Autodesk Fusion 360 part; units mm, degrees
sketch "Sketch1" plane through (0, 0, 0) normal (0, 1, 0) x (1, 0, 0)
  circle A0 centre (0, 0) radius 48 construction
  circle A1 centre (0, 0) radius 14 construction
  circle A2 centre (0, 0) radius 9.5 construction
  circle A3 centre (0, 0) radius 8 construction
  line L0 (0, 0) -> (8, 0) construction
  line L1 (0, 0) -> (0, -9.5) construction
  line L2 (0, 0) -> (-8, 0) construction
  line L3 (0, 0) -> (0, 9.5) construction
  circle A4 centre (8, 0) radius 1.5
  circle A5 centre (-8, 0) radius 1.5
  circle A6 centre (0, 9.5) radius 1.5
  circle A7 centre (0, 0) radius 12 construction
  line L4 (8, 0) -> (18, 0) construction
  line L5 (21.1, 0) -> (19.55, 2.6847) construction
  line L6 (19.55, 2.6847) -> (16.45, 2.6847) construction
  line L7 (16.45, 2.6847) -> (14.9, 0) construction
  line L8 (14.9, 0) -> (16.45, -2.6847) construction
  line L9 (16.45, -2.6847) -> (19.55, -2.6847) construction
  line L10 (19.55, -2.6847) -> (21.1, 0) construction
  circle A8 centre (18, 0) radius 3.1 construction
  circle A9 centre (18, 0) radius 1.5
  line L11 (0, 52) -> (-68, 52) construction
  line L12 (-9.7468, 47) -> (-68, 47) construction
  line L13 (-68, 52) -> (-68, 47) construction
  line L14 (-68, 47) -> (-68, 35.633) construction
  line L15 (-68, 35.633) -> (-32.1604, 35.633) construction
  line L16 (-68, 35.633) -> (-68, 30.833) construction
  line L17 (-68, 30.833) -> (-36.7876, 30.833) construction
  line L18 (-68, 30.833) -> (-68, -9.167) construction
  line L19 (-60, -9.167) -> (-47.1165, -9.167)
  line L20 (-68, -9.167) -> (-68, -13.967) construction
  line L21 (-68, -13.967) -> (-45.923, -13.967) construction
  line L22 (-60, -13.967) -> (-60, 35.633)
  line L23 (5.9333, 10.4305) -> (19.5328, 2.6945)
  line L24 (-60, -13.967) -> (21.1, -13.967)
  line L25 (21.1, -13.967) -> (21.1, 0)
  arc A10 (21.1, 0) -> (19.5328, 2.6945) centre (18, 0) ccw
  line L26 (-57, 35.633) -> (5, 35.633)
  line L27 (5, 35.633) -> (5, 11.8322)
  arc A11 (5.9333, 10.4305) -> (5.7778, 10.5175) centre (0, 0) ccw
  arc A12 (5, 11.8322) -> (5.7778, 10.5175) centre (6.5, 11.8322) ccw
  arc A13 (5.7778, 10.5175) -> (7.9656, 11.513) centre (6.5, 11.8322) ccw construction
  arc A14 (5.4445, 12.898) -> (5, 11.8322) centre (6.5, 11.8322) ccw construction
  arc A15 (7.9656, 11.513) -> (5.4445, 12.898) centre (6.5, 11.8322) ccw construction
  line L28 (5, 11.8322) -> (5, 10.9087) construction
  arc A16 (5.7778, 10.5175) -> (5, 10.9087) centre (0, 0) ccw construction
  line L29 (-57, 30.833) -> (5, 30.833)
  line L30 (-47.1165, -9.167) -> (21.1, -9.167)
  line L31 (-60, 35.633) -> (-60, 45.633)
  line L32 (-60, 45.633) -> (5, 45.633)
  line L33 (5, 45.633) -> (5, 35.633)
  circle A17 centre (-56, 42) radius 1.5
  circle A18 centre (-40, 42) radius 1.5
  line L34 (-40, 42) -> (0, 0) construction
  circle A19 centre (-55.8448, -4.167) radius 1.5
  line L35 (0, 0) -> (-55.8448, -4.167) construction
  line L36 (-68, -9.167) -> (-60, -9.167) construction
  line L37 (-57, -9.167) -> (-60, -8.167)
  line L38 (-57, -9.167) -> (-57, 30.833) construction
  line L39 (-57, 30.833) -> (-57, 35.633) construction
  line L40 (-57, 30.833) -> (-60, 29.833)
  line L41 (-57, 35.633) -> (-60, 36.633)
  line L42 (-60, 35.633) -> (-57, 35.633) construction
  line L43 (-60, 30.833) -> (-57, 30.833) construction
  line L44 (5, 11.8322) -> (5, -13.967) construction
  line L45 (5, -13.967) -> (19.8959, -2.4527)
  line L46 (18, 0) -> (19.8959, -2.4527) construction
  line L47 (18, 0) -> (21.1, 0) construction
  arc A20 (19.8959, -2.4527) -> (21.1, 0) centre (18, 0) ccw
  point P0 (18, 0)
  point P1 (-33.1034, 34.7586)
  point P2 (-47.8669, -3.5717)
  dimension "d1" = 96
  dimension "d2" = 28
  dimension "d3" = 19
  dimension "d4" = 16
  dimension "d5" = 3
  dimension "d6" = 3
  dimension "d7" = 3
  dimension "d8" = 24
  dimension "d9" = 18
  dimension "d10" = 3.1
  dimension "d11" = 60
  dimension "d12" = 3
  dimension "d13" = 52
  dimension "d14" = 68
  dimension "d15" = 68
  dimension "d18" = 5
  dimension "d22" = 16.367
  dimension "d23" = 4.8
  dimension "d24" = 40
  dimension "d25" = 4.8
  dimension "d26" = 8
  dimension "d27" = 3.1
  dimension "d28" = 5
  dimension "d33" = 12
  dimension "d34" = 3
  dimension "d35" = 10
  dimension "d36" = 3
  dimension "d37" = 12
  dimension "d38" = 5
  dimension "d39" = 3
  dimension "d40" = 5
  dimension "d41" = 10
  dimension "d42" = 3
  dimension "d43" = 5
  dimension "d44" = 8
  dimension "d54" = 1
  dimension "d55" = 3
  dimension "d56" = 1
  dimension "d57" = 1
  dimension "d60" = 3.1
extrude "Extrude1" add sketch "Sketch1" along normal blind 4.8 contours L19 L22 L37 | L19 L22 L24 L30 L45 | L19 L22 L23 A10 L27 A11 A12 L29 L30 L37 L40 L45 A20 | L22 L26 L27 L29 L31 L40 L41 | L26 L31 L32 L33 L41 makes body 1
fillet "Fillet1" radius 4 2 edges at (5, 2.4, -45.633) (-60, 2.4, -45.633) on bodies 1
extrude "Extrude2" cut sketch "Sketch1" along normal blind 1.8 contours L19 L22 L37 | L19 L22 L24 L30 L45 | L24 L25 L30 L45 | L22 L26 L27 L29 L31 L40 L41 bodies 1
fillet "Fillet2" radius 3 3 edges at (-57, 0.9, -35.633) (-57, 0.9, -30.833) (-57, 0.9, 9.167) on bodies 1
ref_plane "WorkPlane1" through (-30, 0, 0) normal (1, 0, 0) x (0, 1, 0)
ref_plane "WorkPlane2" through (-25, 0, 0) normal (1, 0, 0) x (0, 1, 0)
split "Split1" by plane through (-30, 0, 0) normal (1, 0, 0) bodies 1 makes body 2 at (-9.9784, 4.8, -33.9796)
split "Split2" by plane through (-25, 0, 0) normal (1, 0, 0) bodies 2 makes body 3 at (-8.25, 4.8, -34.0217)
delete_body "RemoveBody1" bodies 2
move_body "Move1" bodies 3 to x (1, 0, 0) y (0, 1, 0) z (0, 0, 1) at (-5, 0, 0)
combine "Combine1" operation add target body 1 tool bodies 3
Verification items for the finished model (mm, model axes). A direction names the side the tool comes from. Round coordinates to 2 decimals unless told otherwise and drop trailing zeros. Write each loop counter-clockwise with the first axis right and the second up, starting at its lowest first coordinate (ties: lowest second). Pieces come first, ordered by that corner, then holes.
(1) Mould release check, pull along X, two halves, no side actions. Record for faces 5 (the cylindrical face through (11.5, 2.37, 0.07)), 6 (the flat face through (-30, 0, -41)), 7 (the flat face through (-60, 2, -13)), 8 (the cylindrical face through (-1.14, 2.43, -44.43)): pulls with the +X half, pulls with the -X half, needs draft (parallel to the pull), parting line crosses it, or undercut.
Returned:
face 5: undercut
face 6: needs draft
face 7: pulls with the -X half
face 8: pulls with the +X half
(2) Section check C-C (x = -45.5). Enter the section's corners in (y, z), plus the area to 3 significant figures.
Returned:
outline: (0, -45.63) - (4.8, -45.63) - (4.8, 13.97) - (1.8, 13.97) - (1.8, 9.17) - (0, 9.17) - (0, -30.83) - (1.8, -30.83) - (1.8, -35.63) - (0, -35.63) - close
area: 269 mm2
(3) Section check D-D (z = -22.5). Enter the section's corners in (x, y).
Returned:
outline: (-60, 0) - (0, 0) - (0, 4.8) - (-60, 4.8) - close
(4) Access from +Z, -Z, +X, -X, +Y, -Y to the whole of each face (thin tool, end or side, straight path). Record for faces 1 (the flat face through (0, 2, -27)), 2 (the flat face through (-26, 1, 9.167)), 3 (the flat face through (-58.7, 0.9, 8.6)), 4 (the flat face through (-58.713, 0.887, -30.262)).
Returned:
face 1: -Z, +X, +Y, -Y
face 2: +Z, +X, -X, -Y
face 3: +Z, -X, -Y
face 4: -X, -Y
(5) Section check A-A (y = 1). Give the number of separate pieces and of enclosed holes in the cut face, plus the area to 3 significant figures.
Returned:
separate pieces: 2
enclosed holes: 7
area: 3,150 mm2
(6) Section check B-B (x = -5). Enter the section's corners in (y, z), plus the area to 3 significant figures.
Returned:
outline: (0, -45.63) - (4.8, -45.63) - (4.8, -11) - (0, -11) - (0, -30.83) - (1.8, -30.83) - (1.8, -35.63) - (0, -35.63) - close; (0, -8) - (4.8, -8) - (4.8, 13.97) - (1.8, 13.97) - (1.8, 9.17) - (0, 9.17) - close
area: 254 mm2
(7) Material ranges on line 1 (X direction, y = 2.35, z = 0); line 2 (Z direction, x = -56, y = 2.15); line 3 (X direction, y = 3.3, z = -42), recorded low to high.
Returned:
line 1: x = -60 to -14.5, -11.5 to 1.5, 4.5 to 11.5, 14.5 to 16.1
line 2: z = -45.63 to -43.5, -40.5 to 2.68, 5.66 to 13.97
line 3: x = -59.98 to -57.5, -54.5 to -41.5, -38.5 to -0.02
(8) Depth check by flat-ended pin: pin 1 Ø2.5 at (y, z) = (3, -27.5) entering from +X; pin 2 Ø2 at (x, y) = (4.5, 0.5) entering from -Z; pin 3 Ø4.5 at (x, z) = (-16, 11.5) entering from -Y; pin 4 Ø2.5 at (x, z) = (-56, -42) entering from +Y. Enter the tip coordinate at first touch or a pass-through.
Returned:
pin 1: stops at x = 0
pin 2: stops at z = -8.97
pin 3: stops at y = 1.8
pin 4: passes through
